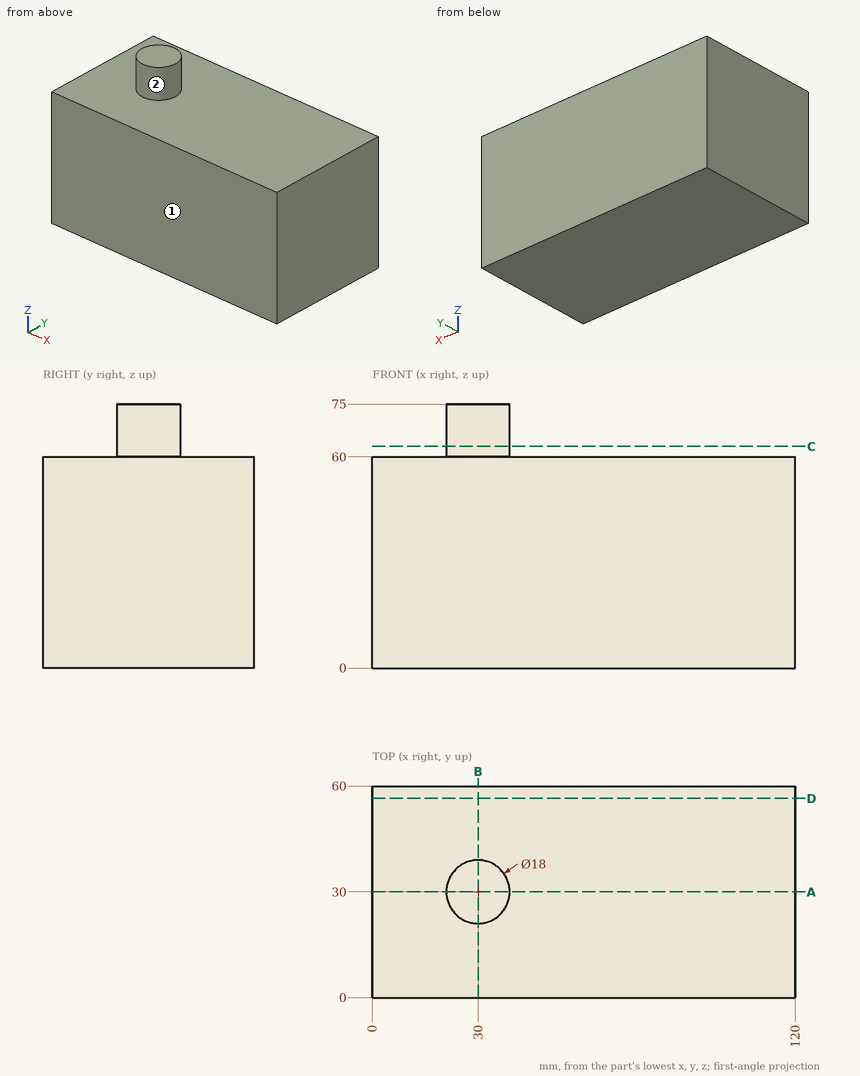
Input: dimensioned drawing with shaded views. Units: mm. Origin: part minimum x, y, z. A direction names the side the tool comes from. Coordinates: 2 decimals unless noted, no trailing zeros. Order: outer loops, then holes, each group sorted by start corner. A loop starts at its lowest first (then second) coordinate and runs counter-clockwise, first axis right, second up. Notation, with made-up numbers: (10.5, 51) - (57.5, 51) arc R16 cw to (57.5, 66) - close; hole circle Ø7 at (16, 0). An arc over 180 degrees is marked (long way). Return JSON: item names as keys, results as strings. Group by question number.
1. Pin query (flat end, axial travel): pin 1 (5 mm diameter, centred on x = 78.5, y = 42.5, fed in from +Z); pin 2 (10 mm diameter, centred on x = 79, z = 63.5, fed in from -Y); pin 3 (4 mm diameter, centred on y = 7.5, z = 63, fed in from +X). Return the tip coordinate at first contact, or that it passes through.
2. Cut plane D-D (y = 56.5). Output: boundary loops of the cut face in (x, z), plus the area to 3 significant figures.
3. Cut plane B-B (x = 30). Output: boundary loops of the cut face in (y, z).
4. Cut plane C-C (z = 63). Output: boundary loops of the cut face in (x, y), plus the area to 3 significant figures.
5. Material intervals for line 1 along Z through (x, y) = (6.5, 24), sorted ascending. Write a range as [from, to].
6. Cut plane A-A (y = 30). Output: boundary loops of the cut face in (x, z).
7. Set-up query: the marked faces 1 and 2. Return all of +Z, -Z, +X, -X, +Y, -Y with unobstructed straight access to the full face (end or side cutting, diameter ignored); none if empty.
Resolved:
{
 "1": {"pin 1": "stops at z = 60", "pin 2": "stops at y = 0", "pin 3": "passes through"},
 "2": {"outline": "(0, 0) - (120, 0) - (120, 60) - (0, 60) - close", "area": "7,200 mm²"},
 "3": {"outline": "(0, 0) - (60, 0) - (60, 60) - (39, 60) - (39, 75) - (21, 75) - (21, 60) - (0, 60) - close"},
 "4": {"outline": "circle Ø18 at (30, 30)", "area": "254 mm²"},
 "5": {"line 1": "z = [0, 60]"},
 "6": {"outline": "(0, 0) - (120, 0) - (120, 60) - (39, 60) - (39, 75) - (21, 75) - (21, 60) - (0, 60) - close"},
 "7": {"face 1": "+Z, -Z, +X, -X, -Y", "face 2": "+Z"}
}
